from build123d import *

# Parameters (mm, degrees)
F0_W     = 31.5
F0_H     = 12.5
F0_R     = 3.25
F0_R_2   = 2.5
F1_DEPTH = 25
F2_T     = -1.2
F3_R     = 3.25
F3_R_2   = 2.5
F4_DEPTH = 4
F5_DEPTH = 25
F6_DEPTH = 8
F7_DEPTH = 4
F8_R     = 2


# Not quite as in the source:
# - a fillet or chamfer that OpenCascade refuses, or shapes differently, is made with other operations: its cross-section is extruded or revolved along the edge and cut away or added


with BuildPart() as f1:
    # F0 (on Front) → F1 (new body)
    with BuildSketch(Plane.XZ):
        with Locations((-14.899123773, 20.1096497476)):
            Rectangle(F0_W, F0_H)
        with Locations((-24.399123773, 20.1096497476)):
            Circle(F0_R, mode=Mode.SUBTRACT)
        with Locations((-14.899123773, 20.1096497476)):
            Circle(F0_R, mode=Mode.SUBTRACT)
        with Locations((-5.399123773, 20.1096497476)):
            Circle(F0_R, mode=Mode.SUBTRACT)
        with Locations((-5.399123773, 20.1096497476)):
            Circle(F0_R)
        with Locations((-5.399123773, 20.1096497476)):
            Circle(F0_R_2, mode=Mode.SUBTRACT)
        with Locations((-14.899123773, 20.1096497476)):
            Circle(F0_R)
        with Locations((-14.899123773, 20.1096497476)):
            Circle(F0_R_2, mode=Mode.SUBTRACT)
        with Locations((-24.399123773, 20.1096497476)):
            Circle(F0_R)
        with Locations((-24.399123773, 20.1096497476)):
            Circle(F0_R_2, mode=Mode.SUBTRACT)
        with Locations((-5.399123773, 20.1096497476)):
            Circle(F0_R_2)
        with Locations((-14.899123773, 20.1096497476)):
            Circle(F0_R_2)
        with Locations((-24.399123773, 20.1096497476)):
            Circle(F0_R_2)
    extrude(amount=-F1_DEPTH)

    # F2
    f2_openings = [f1.faces().sort_by_distance(p)[0] for p in [
        (-14.899124, 12.5, 26.35965),
    ]]
    offset(amount=F2_T, openings=f2_openings)

    # F3 (on face) → F4 (join)
    with BuildSketch(Plane(origin=(0, 25, 0), x_dir=(-1, 0, 0), z_dir=(0, 1, 0))):
        with Locations((14.9896983057, 20.05478926)):
            Circle(F3_R)
        with Locations((14.9896983057, 20.05478926)):
            Circle(F3_R_2, mode=Mode.SUBTRACT)
    extrude(amount=F4_DEPTH)

    # F5 (cut): a face of the model
    f5_faces = [f1.faces().sort_by_distance(p)[0] for p in [
        (-14.9896983057, 25, 20.05478926),
    ]]
    extrude(f5_faces, amount=-F5_DEPTH, mode=Mode.SUBTRACT)

    # F0 (on Front) → F6 (cut)
    with BuildSketch(Plane.XZ):
        with Locations((-24.399123773, 20.1096497476)):
            Circle(F0_R_2)
        with Locations((-5.399123773, 20.1096497476)):
            Circle(F0_R_2)
    extrude(amount=-F6_DEPTH, mode=Mode.SUBTRACT)

    # F0 (on Front) → F7 (join)
    with BuildSketch(Plane.XZ):
        with Locations((-24.399123773, 20.1096497476)):
            Circle(F0_R)
        with Locations((-24.399123773, 20.1096497476)):
            Circle(F0_R_2, mode=Mode.SUBTRACT)
        with Locations((-14.899123773, 20.1096497476)):
            Circle(F0_R)
        with Locations((-14.899123773, 20.1096497476)):
            Circle(F0_R_2, mode=Mode.SUBTRACT)
        with Locations((-5.399123773, 20.1096497476)):
            Circle(F0_R)
        with Locations((-5.399123773, 20.1096497476)):
            Circle(F0_R_2, mode=Mode.SUBTRACT)
    extrude(amount=F7_DEPTH)

    # F8
    f8_edges = [f1.edges().sort_by_distance(p)[0] for p in [
        (0.850876, 12.5, 13.85965),
        (0.850876, 0, 20.10965),
        (-14.899124, 0, 13.85965),
        (-30.649124, 12.5, 13.85965),
        (-30.649124, 0, 20.10965),
        (-30.649124, 25, 20.10965),
        (-14.899124, 25, 13.85965),
        (0.850876, 25, 20.10965),
    ]]
    fillet(f8_edges, radius=F8_R)

    # F9: fillet of radius 1 on 4 edges, made by hand

    # F9_s1 → F9_t2 (revolve, cut)
    with BuildSketch(Plane.XY.offset(20.1096497476)):
        with BuildLine():
            ThreePointArc((-2.148723773, -3.0310064355), (-2.3582112834, -3.6439193102), (-2.8990234836, -4.0003872235))
            Line((-2.8990234836, -4.0003872235), (-2.8739168861, -4.0973253023))
            ThreePointArc((-2.8739168861, -4.0973253023), (-2.5240736283, -4.1001365685), (-2.149123773, -4.1001365685))
            Line((-2.149123773, -4.1001365685), (-2.0489872044, -4))
            ThreePointArc((-2.0489872044, -4), (-2.0489872044, -3.5155032177), (-2.0485872044, -3.0310064355))
            Line((-2.0485872044, -3.0310064355), (-2.148723773, -3.0310064355))
        make_face()
    revolve(axis=Axis((-5.399123773, -4, 20.1096497476), (0, -1, 0)), mode=Mode.SUBTRACT)

    # F9_s3 → F9_t4 (revolve, cut)
    with BuildSketch(Plane.XY.offset(20.1096497476)):
        with BuildLine():
            ThreePointArc((-11.648723773, -3.0310064355), (-11.8582112834, -3.6439193102), (-12.3990234836, -4.0003872235))
            Line((-12.3990234836, -4.0003872235), (-12.3739168861, -4.0973253023))
            ThreePointArc((-12.3739168861, -4.0973253023), (-12.0240736283, -4.1001365685), (-11.649123773, -4.1001365685))
            Line((-11.649123773, -4.1001365685), (-11.5489872044, -4))
            ThreePointArc((-11.5489872044, -4), (-11.5489872044, -3.5155032177), (-11.5485872044, -3.0310064355))
            Line((-11.5485872044, -3.0310064355), (-11.648723773, -3.0310064355))
        make_face()
    revolve(axis=Axis((-14.899123773, -4, 20.1096497476), (0, -1, 0)), mode=Mode.SUBTRACT)

    # F9_s5 → F9_t6 (revolve, cut)
    with BuildSketch(Plane.XY.offset(20.1096497476)):
        with BuildLine():
            ThreePointArc((-21.148723773, -3.0310064355), (-21.3582112834, -3.6439193102), (-21.8990234836, -4.0003872235))
            Line((-21.8990234836, -4.0003872235), (-21.8739168861, -4.0973253023))
            ThreePointArc((-21.8739168861, -4.0973253023), (-21.5240736283, -4.1001365685), (-21.149123773, -4.1001365685))
            Line((-21.149123773, -4.1001365685), (-21.0489872044, -4))
            ThreePointArc((-21.0489872044, -4), (-21.0489872044, -3.5155032177), (-21.0485872044, -3.0310064355))
            Line((-21.0485872044, -3.0310064355), (-21.148723773, -3.0310064355))
        make_face()
    revolve(axis=Axis((-24.399123773, -4, 20.1096497476), (0, -1, 0)), mode=Mode.SUBTRACT)

    # F9_s7 → F9_t8 (revolve, cut)
    with BuildSketch(Plane.XY.offset(20.05478926)):
        with BuildLine():
            ThreePointArc((-18.2400983057, 28.0310064355), (-18.0306107953, 28.6439193102), (-17.4897985952, 29.0003872235))
            Line((-17.4897985952, 29.0003872235), (-17.5149051926, 29.0973253023))
            ThreePointArc((-17.5149051926, 29.0973253023), (-17.8647484504, 29.1001365685), (-18.2396983057, 29.1001365685))
            Line((-18.2396983057, 29.1001365685), (-18.3398348743, 29))
            ThreePointArc((-18.3398348743, 29), (-18.3398348743, 28.5155032177), (-18.3402348743, 28.0310064355))
            Line((-18.3402348743, 28.0310064355), (-18.2400983057, 28.0310064355))
        make_face()
    revolve(axis=Axis((-14.9896983057, 29, 20.05478926), (0, 1, 0)), mode=Mode.SUBTRACT)


solid = f1.part
Model file for the job. Use its own axes, mm. A direction names the side the tool comes from. Coordinates: 2 decimals unless noted, no trailing zeros. Write each loop counter-clockwise with the first axis right and the second up, starting at its lowest first coordinate (ties: lowest second). Pieces come first, ordered by that corner, then holes. Notation, with made-up numbers: (-36.5, -14.5) -> (6.5, -14.5) arc R32 ccw to (6.5, 12.5) -> close; hole circle Ø4 at (29.25, -11.5). An arc over 180 degrees is marked (long way). One line per item, written item: value. Start each with the question number.
1) Which spindle directions (+Z, -Z, +X, -X, +Y, -Y) get a long thin tool onto all of the face, cutting with end or side? Do faces 1 (the face through (-12.515, -1.972, 20.861)), 2 (the face through (-15, 12, 13.86)), 3 (the face through (-29.449, 12, 21)). Say none if no direction does.
2) Slice it at C-C on x = -19.5. Write the cut outline in (y, z).
3) Flat gauge pins, fed straight in: pin 1 Ø3 at (x, z) = (-14.5, 16) entering from +Y; pin 2 Ø2 at (x, z) = (-3, 17) entering from -Y; pin 3 Ø7 at (x, y) = (-17, 9) entering from +Z. Where does each tip first touch, or does it go through?
4) Slice it at B-B on y = 16.5. Write the cut outline in (x, z).
5) Slice it at D-D on y = 0.5. Write the cut outline in (x, z), then the cut area to 3 significant figures.
6) Slice it at A-A on z = 25.75. Write the cut outline in (x, y).
7) Pull direction X, two halves, no side cores. Call faces 4 (the face through (-15, 1.2, 23)), 5 (the face through (-18.1, 26.5, 21)), 6 (the face through (-15, 23.8, 23)), 7 (the face through (-30.05, 0.57, 21.18)): +X half, -X half, draft (parallel to the pull), parting line (faces both ways), or undercut.
8) Probe probe 1 along Y at (x, z) = (-3, 16.5); probe 2 along X at (y, z) = (3, 18.75); probe 3 along Z at (x, y) = (-26, 17.5). List the from-to ranges inside material, lowest first.
Answers follow:
1. face 1: -Y
1. face 2: -Z, +X, -X, +Y, -Y
1. face 3: +Z
2. outline: (0, 15.86) arc R2 ccw to (2, 13.86) -> (23, 13.86) arc R2 ccw to (25, 15.86) -> (25, 26.36) -> (23.8, 26.36) -> (23.8, 15.06) -> (1.2, 15.06) -> (1.2, 26.36) -> (0, 26.36) -> close
3. pin 1: y = 28.97
3. pin 2: y = -3.77
3. pin 3: z = 15.06
4. outline: (-30.65, 15.86) arc R2 ccw to (-28.65, 13.86) -> (-1.15, 13.86) arc R2 ccw to (0.85, 15.86) -> (0.85, 26.36) -> (-0.35, 26.36) -> (-0.35, 15.06) -> (-29.45, 15.06) -> (-29.45, 26.36) -> (-30.65, 26.36) -> close
5. outline: (-29.97, 15.86) arc R1.32 ccw to (-28.65, 14.54) -> (-1.15, 14.54) arc R1.32 ccw to (0.17, 15.86) -> (0.17, 26.36) -> (-29.97, 26.36) -> close; hole circle Ø5 at (-24.4, 20.11); hole circle Ø5 at (-14.99, 20.05); hole circle Ø5 at (-5.4, 20.11)
5. area: 297 mm2
6. outline: (-30.65, 2) arc R2 ccw to (-28.65, 0) -> (-1.15, 0) arc R2 ccw to (0.85, 2) -> (0.85, 23) arc R2 ccw to (-1.15, 25) -> (-28.65, 25) arc R2 ccw to (-30.65, 23) -> close; hole (-29.45, 1.2) -> (-0.35, 1.2) -> (-0.35, 23.8) -> (-29.45, 23.8) -> close
7. face 4: undercut
7. face 5: parting line
7. face 6: undercut
7. face 7: -X half
8. probe 1: 0 to 1.2, 23.8 to 25
8. probe 2: -30.65 to -29.45, -0.35 to 0.85
8. probe 3: 13.86 to 15.06
